Design review of the part shown in the three views and the two pictorial views. Dimensions are in mm from the part's minimum x, y and z. Coordinates: 2 decimals unless noted, no trailing zeros. Loops run counter-clockwise (first coordinate to the right, second up) from the corner with the lowest first, then second, coordinate; pieces in that order, holes last. Notation, with made-up numbers: (38.5, 16.5) - (90.5, 16.5) arc R7 cw to (90.5, 23.5) - close; hole circle Ø6 at (56, 19). An arc over 180 degrees is marked (long way). One line per item, written item: value. Start each with the question number.
1. Take a section at C-C, the plane y = 14.5. State the section outline as (x, z) points, and give its area (3 significant figures).
2. The part is to be moulded in two halves that separate along X. For the marked faces 1, 2, 3 and 4, say which applies: released by +X, released by -X, zero draft, split by the parting line, or undercut.
3. To check wall thickness, follow line 1 (Y direction, x = 4.5, z = 1.95); line 2 (Y direction, x = 2.3, z = 2.05); line 3 (X direction, y = 47, z = 0.75). State the ranges of each line that lie inside material, in increasing order. Write a range as from..to.
4. Take a section at A-A, the plane x = 2.8. State the section outline as (y, z) points.
5. Insertion check: pin 1 (2 mm diameter, centred on y = 24, z = 2, fed in from +X). The pin has a flat end and moves straight along its axis. Give the tip position at first contact, or say it passes through.
6. Take a section at B-B, the plane z = 2. State the section outline as (x, y) points, and give its area (3 significant figures).
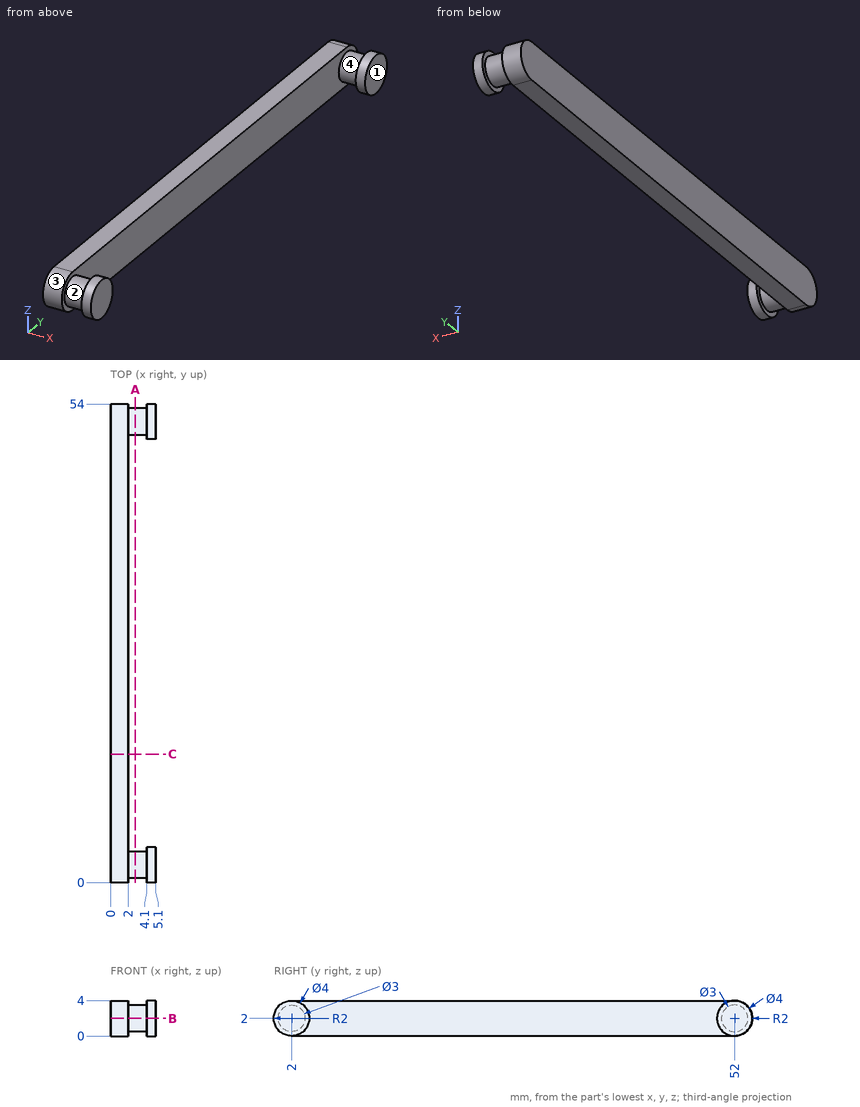
Solutions:
1. outline: (0, 0) - (2, 0) - (2, 4) - (0, 4) - close
1. area: 8.00 mm2
2. face 1: released by +X
2. face 2: undercut
2. face 3: zero draft
2. face 4: undercut
3. line 1: 0..4, 50..54
3. line 2: 0.5..3.5, 50.5..53.5
3. line 3: 0..2
4. outline: circle Ø3 at (2, 2); circle Ø3 at (52, 2)
5. pin 1: x = 2
6. outline: (0, 0) - (2, 0) - (2, 0.5) - (4.1, 0.5) - (4.1, 0) - (5.1, 0) - (5.1, 4) - (4.1, 4) - (4.1, 3.5) - (2, 3.5) - (2, 50.5) - (4.1, 50.5) - (4.1, 50) - (5.1, 50) - (5.1, 54) - (4.1, 54) - (4.1, 53.5) - (2, 53.5) - (2, 54) - (0, 54) - close
6. area: 129 mm2
